```python
from build123d import *

# Parameters (mm, degrees)
CROQUIS1_R              = 6
SALIENTE_EXTRUIR1_DEPTH = 5
REDONDEO1_R             = 10
REDONDEO3_R             = 10
CROQUIS2_R              = 50
CROQUIS2_R_2            = 41
SALIENTE_EXTRUIR3_DEPTH = 10
CROQUIS3_W              = 20
CROQUIS3_H              = 40.5
CORTAR_EXTRUIR1_DEPTH   = 10
CORTAR_EXTRUIR2_DEPTH   = 10
CROQUIS5_R              = 50
SALIENTE_EXTRUIR4_DEPTH = 10


with BuildPart() as part:
    # Croquis1 → Saliente-Extruir1 (new body)
    with BuildSketch(Plane.XY):
        with BuildLine():
            ThreePointArc((50, 164), (0, 214), (-50, 164))
            Line((-50, 164), (-50, 11.739233328))
            Line((-50, 11.739233328), (-20, 0))
            Line((-20, 0), (-13.787308542, -2.431074487))
            add(Edge.make_bspline(
                [(-8.854817181, -5.677302066), (-9.51760475, -5.090344722), (-10.900654261, -3.469047842), (-12.711160318, -2.852179657), (-13.787308542, -2.431074487)],
                knots=[0.517708821, 0.517708821, 0.517708821, 0.517708821, 0.741171884, 1, 1, 1, 1], degree=3))
            ThreePointArc((-8.854817181, -5.677302066), (0, -9.578400122), (8.854817181, -5.677302066))
            add(Edge.make_bspline(
                [(8.854817181, -5.677302066), (9.51760475, -5.090344722), (10.900654261, -3.469047842), (12.711160318, -2.852179657), (13.787308542, -2.431074487)],
                knots=[0.517708821, 0.517708821, 0.517708821, 0.517708821, 0.741171884, 1, 1, 1, 1], degree=3))
            Line((13.787308542, -2.431074487), (20, 0))
            Line((20, 0), (50, 11.739233328))
            Line((50, 11.739233328), (50, 164))
        make_face()
        Circle(CROQUIS1_R, mode=Mode.SUBTRACT)
    extrude(amount=SALIENTE_EXTRUIR1_DEPTH)

    # Redondeo1
    redondeo1_edges = [part.edges().sort_by_distance(p)[0] for p in [
        (50, 11.739233328, 2.5),
    ]]
    fillet(redondeo1_edges, radius=REDONDEO1_R)

    # Redondeo3
    redondeo3_edges = [part.edges().sort_by_distance(p)[0] for p in [
        (-50, 11.739233328, 2.5),
    ]]
    fillet(redondeo3_edges, radius=REDONDEO3_R)

    # Croquis2 → Saliente-Extruir3 (add)
    with BuildSketch(Plane.XY.offset(5)):
        with Locations((0, 164)):
            Circle(CROQUIS2_R)
        with Locations((0, 164)):
            Circle(CROQUIS2_R_2, mode=Mode.SUBTRACT)
    extrude(amount=SALIENTE_EXTRUIR3_DEPTH)

    # Croquis3 → Cortar-Extruir1 (cut)
    with BuildSketch(Plane(origin=(0, 0, 0), x_dir=(-1, 0, 0), z_dir=(0, 0, -1))):
        with Locations((0, 153.891101056)):
            Rectangle(CROQUIS3_W, CROQUIS3_H)
    extrude(amount=-CORTAR_EXTRUIR1_DEPTH, mode=Mode.SUBTRACT)

    # Croquis4 → Cortar-Extruir2 (cut)
    with BuildSketch(Plane.XY.offset(15)):
        with BuildLine():
            Line((-41, 164), (-50, 164))
            ThreePointArc((-50, 164), (0, 114), (50, 164))
            Line((50, 164), (41, 164))
            ThreePointArc((41, 164), (0, 123), (-41, 164))
        make_face()
    extrude(amount=-CORTAR_EXTRUIR2_DEPTH, mode=Mode.SUBTRACT)

    # Croquis5 → Saliente-Extruir4 (add)
    with BuildSketch(Plane(origin=(0, 0, 0), x_dir=(-1, 0, 0), z_dir=(0, 0, -1))):
        with Locations((0, 164)):
            Circle(CROQUIS5_R)
        Polygon((-10, 174.141101056), (-8, 174.141101056), (-8, 194.141101056), (8, 194.141101056), (8, 174.141101056), (10, 174.141101056), (10, 133.641101056), (-10, 133.641101056), align=None, mode=Mode.SUBTRACT)
    extrude(amount=SALIENTE_EXTRUIR4_DEPTH)


solid = part.part
```
Work out the finished part from the listing and answer in its coordinate system (mm). A direction names the side the tool comes from. Give positions to 0.01 mm unless a question says otherwise; leave off trailing zeros. Order: outer loops, then holes, each group sorted by start corner. A loop starts at its lowest first (then second) coordinate and runs counter-clockwise, first axis right, second up. Notation, with made-up numbers: (1.25, -17.5) -> (9.25, -17.5) arc R15 cw to (9.25, 7.5) -> close; hole circle Ø3 at (-25, 32.5). An arc over 180 degrees is marked (long way). Answer as CSV lines item,"result". Start each with the question number.
(1) Section C-C, the plane x = 16 is taken. Write down the section's boundary in (y, z).
(2) Which of the six approach directions +Z, -Z, +X, -X, +Y, -Y give full straight-line access (tool end or side, diameter ignored) to faces 1 (the flat face through (-8, 184, -5)), 2 (the cylindrical face through (0.9, 204.99, 9.93)), 3 (the flat face through (-45, 164, 10))?
(3) Each of these flat-tipped pins is pushed along its axis until it touches: pin 1 Ø5 at (x, y) = (-4, 108) entering from +Z; pin 2 Ø8 at (x, z) = (1, 10) entering from -Y; pin 3 Ø3 at (x, z) = (1, -5) entering from -Y. Where does it stop, or does it pass through?
(4) Section D-D, the plane z = 12.75 is taken. Write down the section's boundary in (x, y).
(5) For a pull along Y with two mould halves and no side action, classify faces 4 (the flat face through (46, 164, 10)), 5 (the flat face through (8, 184, -5)), 6 (the flat face through (-50, 92, 2)) as released by +Y, released by -Y, zero draft, split by the parting line, or undercut.
(6) Consider line 1 along Y through (x, z) = (0, 2.95); line 2 along Z through (x, y) = (21, 4); line 3 along X through (y, z) = (167, 10.75). Determine where each line is inside the solid, lowest interval first.
(7) Section A-A, the plane x = 0 is taken. Write down the section's boundary in (y, z).
(8) Section B-B, the plane y = 127 is taken. Write down the section's boundary in (x, z), plus the area to 3 significant figures.
Entries:
1,outline,"(-1.57, 0) -> (116.63, 0) -> (116.63, -10) -> (211.37, -10) -> (211.37, 15) -> (201.75, 15) -> (201.75, 5) -> (-1.57, 5) -> close"
2,face 1,"-Z"
2,face 2,"+Z, -Y"
2,face 3,"+Z, +X, -X, -Y"
3,pin 1,"z = 5"
3,pin 2,"y = 204.69"
3,pin 3,"y = 114"
4,outline,"(-50, 164) -> (-41, 164) arc R41 cw to (41, 164) -> (50, 164) arc R50 ccw to start"
5,face 4,"released by -Y"
5,face 5,"undercut"
5,face 6,"zero draft"
6,line 1,"-9.58 to -6, 6 to 133.64, 174.14 to 214"
6,line 2,"0 to 5"
6,line 3,"-49.91 to -40.89, 40.89 to 49.91"
7,outline,"(-9.58, 0) -> (-6, 0) -> (-6, 5) -> (-9.58, 5) -> close; (6, 0) -> (114, 0) -> (114, -10) -> (133.64, -10) -> (133.64, 5) -> (6, 5) -> close; (174.14, 0) -> (194.14, 0) -> (194.14, -10) -> (214, -10) -> (214, 15) -> (205, 15) -> (205, 5) -> (174.14, 5) -> close"
8,outline,"(-50, 0) -> (-33.63, 0) -> (-33.63, -10) -> (33.63, -10) -> (33.63, 0) -> (50, 0) -> (50, 5) -> (-50, 5) -> close"
8,area,"1,170 mm²"
